Build history of the part. All positions in model axes, mm. A direction names the side the tool comes from. Round coordinates to 2 decimals unless told otherwise and drop trailing zeros. Order: outer loops, then holes, each group sorted by start corner. A loop starts at its lowest first (then second) coordinate and runs counter-clockwise, first axis right, second up. Notation, with made-up numbers: (70.25, 66) -> (124.25, 66) arc R15 ccw to (124.25, 95) -> close; hole circle Ø8 at (-9.75, -38). An arc over 180 degrees is marked (long way). Answer as a JSON object with one key per item and string values.
from build123d import *

# Parameters (mm, degrees)
F0_R     = 0.636476
F1_DEPTH = 130


with BuildPart() as f1:
    # F0 (on Front) → F1 (new body)
    with BuildSketch(Plane.XZ):
        Polygon((-12.308648, 30.563487), (-86.652653, 20.890858), (-86.652653, 10.133532), (73.347347, 10.133532), (42.023724, 30.563487), (12.39394, 30.563487), align=None)
        with BuildLine():
            ThreePointArc((-19.014622, 41.418116), (-19.166356, 33.82559), (-12.308648, 30.563487))
            Line((-12.308648, 30.563487), (12.39394, 30.563487))
            Line((12.39394, 30.563487), (17.338732, 33.726226))
            Line((17.338732, 33.726226), (17.338732, 36.697887))
            Line((17.338732, 36.697887), (17.338732, 39.282866))
            Line((17.338732, 39.282866), (17.338732, 41.418116))
            Line((17.338732, 41.418116), (12.39394, 43.066382))
            Line((12.39394, 43.066382), (-15.351817, 43.066382))
            Line((-15.351817, 43.066382), (-19.014622, 41.418116))
        make_face()
        Polygon((17.338732, 39.282866), (17.338732, 36.697887), (58.978832, 36.697887), (58.978832, 37.299656), (58.978832, 38.788896), (58.978832, 39.282866), align=None)
        with BuildLine():
            Line((58.978832, 37.299656), (58.978832, 36.697887))
            Line((58.978832, 36.697887), (60.444385, 35.799279))
            Line((60.444385, 35.799279), (65.389156, 35.799279))
            Line((65.389156, 35.799279), (66.625345, 36.697887))
            Line((66.625345, 36.697887), (66.625345, 39.341377))
            Line((66.625345, 39.341377), (65.389156, 40.057271))
            Line((65.389156, 40.057271), (60.444385, 40.057271))
            Line((60.444385, 40.057271), (58.978832, 39.282866))
            Line((58.978832, 39.282866), (58.978832, 38.788896))
            ThreePointArc((58.978832, 38.788896), (59.421711, 38.044276), (58.978832, 37.299656))
        make_face()
        with Locations((62.932795, 38.143512)):
            Circle(F0_R, mode=Mode.SUBTRACT)
    extrude(amount=F1_DEPTH)


solid = f1.part
1) Probe L1, parallel to X at y = -118, z = 38; L2, parallel to Z at x = 39, y = -48; L3, parallel to X at y = -97, z = 38.5. List the from-to ranges inside material, lowest first. Write a range as from..to.
Checked values:
{"L1": "x = -20.19..58.98, 59.42..62.31, 63.55..66.63", "L2": "z = 10.13..30.56, 36.7..39.28", "L3": "x = -20.14..58.98, 59.29..62.41, 63.46..66.63"}
2) Cut at D-D, the plane z = 17. Give the cut face in (x, y), plus the area to 3 significant figures.
Checked values:
{"outline": "(-86.65, -130) -> (62.82, -130) -> (62.82, 0) -> (-86.65, 0) -> close", "area": "19,400 mm²"}
3) Cut at A-A, the plane x = 54.5. Give the cut face in (y, z), plus the area to 3 significant figures.
Checked values:
{"outline": "(-130, 10.13) -> (0, 10.13) -> (0, 22.43) -> (-130, 22.43) -> close; (-130, 36.7) -> (0, 36.7) -> (0, 39.28) -> (-130, 39.28) -> close", "area": "1,930 mm²"}
4) Pull direction Z, two halves, no side cores. Call faces 1 (the face through (63, -64, 35.799)), 2 (the face through (-8, -64, 10.134)), 3 (the face through (-86.653, -64, 16)): pulls with the +Z half, pulls with the -Z half, needs draft (parallel to the pull), parting line crosses it, or undercut.
Checked values:
{"face 1": "undercut", "face 2": "pulls with the -Z half", "face 3": "needs draft"}
5) Cut at B-B, the plane y = -101.5. Give the cut face in (x, z).
Checked values:
{"outline": "(-86.65, 10.13) -> (73.35, 10.13) -> (42.02, 30.56) -> (12.39, 30.56) -> (17.34, 33.73) -> (17.34, 36.7) -> (58.98, 36.7) -> (60.44, 35.8) -> (65.39, 35.8) -> (66.63, 36.7) -> (66.63, 39.34) -> (65.39, 40.06) -> (60.44, 40.06) -> (58.98, 39.28) -> (17.34, 39.28) -> (17.34, 41.42) -> (12.39, 43.07) -> (-15.35, 43.07) -> (-19.01, 41.42) arc R7 ccw to (-12.31, 30.56) -> (-86.65, 20.89) -> close; hole (58.98, 37.3) arc R0.85 ccw to (58.98, 38.79) -> close; hole circle Ø1.27 at (62.93, 38.14)"}
6) Cut at C-C, the plane x = 33. Give the cut face in (y, z), plus the area to 3 significant figures.
Checked values:
{"outline": "(-130, 10.13) -> (0, 10.13) -> (0, 30.56) -> (-130, 30.56) -> close; (-130, 36.7) -> (0, 36.7) -> (0, 39.28) -> (-130, 39.28) -> close", "area": "2,990 mm²"}
7) Flat gauge pins, fed straight in: pin 1 Ø3 at (y, z) = (-78.5, 28) entering from +X; pin 2 Ø8 at (x, z) = (30, 34.5) entering from -Y; pin 3 Ø1.5 at (y, z) = (-46, 14.5) entering from +X; pin 4 Ø1.2 at (y, z) = (-92, 38) entering from +X. Where does each tip first touch, or does it go through?
Checked values:
{"pin 1": "stops at x = 48.25", "pin 2": "stops at y = -130", "pin 3": "stops at x = 67.8", "pin 4": "stops at x = 66.63"}
8) Which spindle directions (+Z, -Z, +X, -X, +Y, -Y) get a long thin tool onto all of the face, cutting with end or side? Do faces 4 (the face through (63, -64, 40.057)), 5 (the face through (38, -64, 39.283)), 6 (the face through (38, -64, 36.698)). Say none if no direction does.
Checked values:
{"face 4": "+Z, +X, +Y, -Y", "face 5": "+Z, +Y, -Y", "face 6": "+Y, -Y"}
